```python
from build123d import *

# Parameters (mm, degrees)
BOSS_EXTRUDE1_DEPTH = 24
CUT_EXTRUDE1_DEPTH  = 29.5
SKETCH3_R           = 21
BOSS_EXTRUDE2_DEPTH = 24
CUT_EXTRUDE2_DEPTH  = 4
BOSS_EXTRUDE3_DEPTH = 11
SKETCH6_W           = 89
SKETCH6_H           = 21.5
SKETCH7_W           = 48
SKETCH7_H           = 22
BOSS_EXTRUDE4_DEPTH = 3.027047
SKETCH8_R           = 18.5
CUT_EXTRUDE3_DEPTH  = 83
CUT_EXTRUDE4_REACH  = 91
SKETCH9_R           = 1.6
SKETCH9_R_2         = 6.1
CUT_EXTRUDE5_REACH  = 125.5
SKETCH10_R          = 2.9
CUT_EXTRUDE6_REACH  = 136
SKETCH13_R          = 1.9
CUT_EXTRUDE7_DEPTH  = 27


with BuildPart() as part:
    # Sketch1 → Boss-Extrude1 (new body)
    with BuildSketch(Plane(origin=(0, 0, 0), x_dir=(1, 0, 0), z_dir=(0, 1, 0))):
        with BuildLine():
            Line((-42, 0), (-42, 11))
            Line((-42, 11), (-9.786517927, 24.087840644))
            ThreePointArc((-9.786517927, 24.087840644), (26, 0), (-9.786517927, -24.087840644))
            Line((-9.786517927, -24.087840644), (-42, -11))
            Line((-42, -11), (-42, 0))
        make_face()
    extrude(amount=BOSS_EXTRUDE1_DEPTH)

    # Sketch2 → Cut-Extrude1 (cut, symmetric)
    with BuildSketch(Plane.XY):
        Polygon((-24, 0), (26, 12), (26, 0), align=None)
    extrude(amount=CUT_EXTRUDE1_DEPTH, both=True, mode=Mode.SUBTRACT)

    # Sketch3 → Boss-Extrude2 (add)
    with BuildSketch(Plane(origin=(0, 24, 0), x_dir=(1, 0, 0), z_dir=(0, 1, 0))):
        Circle(SKETCH3_R)
    extrude(amount=-BOSS_EXTRUDE2_DEPTH)

    # Sketch4 → Cut-Extrude2 (cut)
    with BuildSketch(Plane.XZ):
        Polygon((2.829016319, 4.9), (-2.829016319, 4.9), (-5.658032638, 0), (-2.829016319, -4.9), (2.829016319, -4.9), (5.658032638, 0), align=None)
    extrude(amount=-CUT_EXTRUDE2_DEPTH, mode=Mode.SUBTRACT)

    # Sketch5 → Boss-Extrude3 (add, symmetric)
    with BuildSketch(Plane.XY):
        with BuildLine():
            ThreePointArc((-54, 24), (-78.945219608, 10.049710337), (-92.941825352, -14.869551102))
            Line((-92.941825352, -14.869551102), (-94.786517927, -22.5))
            Line((-94.786517927, -22.5), (-94.786517927, -37.075307894))
            Line((-94.786517927, -37.075307894), (-93.178015205, -46.5))
            Line((-93.178015205, -46.5), (-90, -56.5))
            Line((-90, -56.5), (-42, -56.5))
            Line((-42, -56.5), (-63.178015205, -46.5))
            Line((-63.178015205, -46.5), (-70.786517927, -37.075307894))
            Line((-70.786517927, -37.075307894), (-70.786517927, -25.075307894))
            Line((-70.786517927, -25.075307894), (-69.738862808, -20.741751748))
            ThreePointArc((-69.738862808, -20.741751748), (-62.647337683, -7.727284744), (-50, 0))
            Line((-50, 0), (-42, 0))
            Line((-42, 0), (-42, 24))
            Line((-42, 24), (-54, 24))
        make_face()
    extrude(amount=BOSS_EXTRUDE3_DEPTH, both=True)



with BuildPart() as body_2:
    # Sketch6 → Revolve1 (revolve)
    with BuildSketch(Plane.XY):
        with Locations((-53.5, -88.75)):
            Rectangle(SKETCH6_W, SKETCH6_H)
    revolve(axis=Axis((-98, -78, 0), (1, 0, 0)))


with BuildPart() as part_1:
    add(part.part)

    add(body_2.part)  # Boss-Extrude4 merges body 2
    # Sketch7 → Boss-Extrude4 (add)
    with BuildSketch(Plane.XZ.offset(56.5)):
        with Locations((-66, 0)):
            Rectangle(SKETCH7_W, SKETCH7_H)
    extrude(amount=BOSS_EXTRUDE4_DEPTH)

    # Sketch8 → Cut-Extrude3 (cut)
    with BuildSketch(Plane.ZY.offset(98)):
        with Locations((0, -78)):
            Circle(SKETCH8_R)
    extrude(amount=-CUT_EXTRUDE3_DEPTH, mode=Mode.SUBTRACT)

    # Sketch9 → Cut-Extrude4 (cut, up to next)
    with BuildSketch(Plane(origin=(-9, 0, 0), x_dir=(0, 0, -1), z_dir=(1, 0, 0)), mode=Mode.PRIVATE) as cut_extrude4_sk1:
        with Locations((15.5, -78)):
            Circle(SKETCH9_R)
    cut_extrude4_tool1 = extrude(cut_extrude4_sk1.sketch, amount=-CUT_EXTRUDE4_REACH, mode=Mode.PRIVATE) & part_1.part
    add(cut_extrude4_tool1.solids().sort_by_distance((-9, -78, -15.5))[0], mode=Mode.SUBTRACT)
    # Sketch9 → Cut-Extrude4 (cut, up to next)
    with BuildSketch(Plane(origin=(-9, 0, 0), x_dir=(0, 0, -1), z_dir=(1, 0, 0)), mode=Mode.PRIVATE) as cut_extrude4_sk2:
        with Locations((7.75, -91.423393759)):
            Circle(SKETCH9_R)
    cut_extrude4_tool2 = extrude(cut_extrude4_sk2.sketch, amount=-CUT_EXTRUDE4_REACH, mode=Mode.PRIVATE) & part_1.part
    add(cut_extrude4_tool2.solids().sort_by_distance((-9, -91.423394, -7.75))[0], mode=Mode.SUBTRACT)
    # Sketch9 → Cut-Extrude4 (cut, up to next)
    with BuildSketch(Plane(origin=(-9, 0, 0), x_dir=(0, 0, -1), z_dir=(1, 0, 0)), mode=Mode.PRIVATE) as cut_extrude4_sk3:
        with Locations((-7.75, -91.423393759)):
            Circle(SKETCH9_R)
    cut_extrude4_tool3 = extrude(cut_extrude4_sk3.sketch, amount=-CUT_EXTRUDE4_REACH, mode=Mode.PRIVATE) & part_1.part
    add(cut_extrude4_tool3.solids().sort_by_distance((-9, -91.423394, 7.75))[0], mode=Mode.SUBTRACT)
    # Sketch9 → Cut-Extrude4 (cut, up to next)
    with BuildSketch(Plane(origin=(-9, 0, 0), x_dir=(0, 0, -1), z_dir=(1, 0, 0)), mode=Mode.PRIVATE) as cut_extrude4_sk4:
        with Locations((-15.5, -78)):
            Circle(SKETCH9_R)
    cut_extrude4_tool4 = extrude(cut_extrude4_sk4.sketch, amount=-CUT_EXTRUDE4_REACH, mode=Mode.PRIVATE) & part_1.part
    add(cut_extrude4_tool4.solids().sort_by_distance((-9, -78, 15.5))[0], mode=Mode.SUBTRACT)
    # Sketch9 → Cut-Extrude4 (cut, up to next)
    with BuildSketch(Plane(origin=(-9, 0, 0), x_dir=(0, 0, -1), z_dir=(1, 0, 0)), mode=Mode.PRIVATE) as cut_extrude4_sk5:
        with Locations((-7.75, -64.576606241)):
            Circle(SKETCH9_R)
    cut_extrude4_tool5 = extrude(cut_extrude4_sk5.sketch, amount=-CUT_EXTRUDE4_REACH, mode=Mode.PRIVATE) & part_1.part
    add(cut_extrude4_tool5.solids().sort_by_distance((-9, -64.576606, 7.75))[0], mode=Mode.SUBTRACT)
    # Sketch9 → Cut-Extrude4 (cut, up to next)
    with BuildSketch(Plane(origin=(-9, 0, 0), x_dir=(0, 0, -1), z_dir=(1, 0, 0)), mode=Mode.PRIVATE) as cut_extrude4_sk6:
        with Locations((7.75, -64.576606241)):
            Circle(SKETCH9_R)
    cut_extrude4_tool6 = extrude(cut_extrude4_sk6.sketch, amount=-CUT_EXTRUDE4_REACH, mode=Mode.PRIVATE) & part_1.part
    add(cut_extrude4_tool6.solids().sort_by_distance((-9, -64.576606, -7.75))[0], mode=Mode.SUBTRACT)
    # Sketch9 → Cut-Extrude4 (cut, up to next)
    with BuildSketch(Plane(origin=(-9, 0, 0), x_dir=(0, 0, -1), z_dir=(1, 0, 0)), mode=Mode.PRIVATE) as cut_extrude4_sk7:
        with Locations((0, -85)):
            Circle(SKETCH9_R_2)
    cut_extrude4_tool7 = extrude(cut_extrude4_sk7.sketch, amount=-CUT_EXTRUDE4_REACH, mode=Mode.PRIVATE) & part_1.part
    add(cut_extrude4_tool7.solids().sort_by_distance((-9, -85, 0))[0], mode=Mode.SUBTRACT)

    # Sketch10 → Cut-Extrude5 (cut, up to next)
    with BuildSketch(Plane(origin=(0, 24, 0), x_dir=(1, 0, 0), z_dir=(0, 1, 0)), mode=Mode.PRIVATE) as cut_extrude5_sk1:
        Circle(SKETCH10_R)
    cut_extrude5_tool1 = extrude(cut_extrude5_sk1.sketch, amount=-CUT_EXTRUDE5_REACH, mode=Mode.PRIVATE) & part_1.part
    add(cut_extrude5_tool1.solids().sort_by_distance((0, 24, 0))[0], mode=Mode.SUBTRACT)

    # Sketch12 → Cut-Extrude6 (cut, up to next)
    with BuildSketch(Plane.ZY.offset(108), mode=Mode.PRIVATE) as cut_extrude6_sk1:
        Polygon((0, -14.869551102), (0, -37.075307894), (-35.009935155, -37.075307894), (-35.009935155, -113.334550455), (34.515095082, -113.334550455), (34.515095082, -14.869551102), align=None)
    cut_extrude6_tool1 = extrude(cut_extrude6_sk1.sketch, amount=-CUT_EXTRUDE6_REACH, mode=Mode.PRIVATE) & part_1.part
    add(cut_extrude6_tool1.solids().sort_by_distance((-108, -68.986865, 1.963457))[0], mode=Mode.SUBTRACT)

    # Sketch13 → Cut-Extrude7 (cut, through all)
    with BuildSketch(Plane.XY):
        with Locations((-81.960177429, -20.369551102)):
            Circle(SKETCH13_R)
        with Locations((-82.786517927, -31.575307894)):
            Circle(SKETCH13_R)
    extrude(amount=-CUT_EXTRUDE7_DEPTH, mode=Mode.SUBTRACT)


solid = part_1.part
```
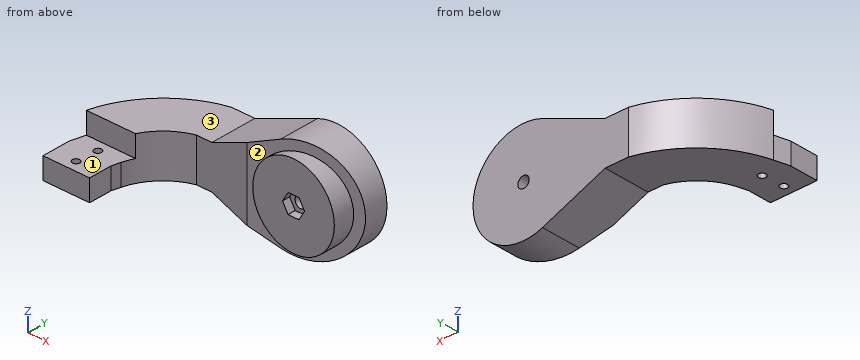
Could you check a few things on this model? Use its own coordinates, in mm. Face numbers are marked on the shaded views. A direction names the side the tool comes from. Round coordinates to 2 decimals unless told otherwise and drop trailing zeros. Loops run counter-clockwise (first coordinate to the right, second up) from the corner with the lowest first, then second, coordinate; pieces in that order, holes last. Notation, with made-up numbers: (34, 79) - (78, 79) arc R24 cw to (78, 112) - close; hole circle Ø9 at (38, 42). An arc over 180 degrees is marked (long way). Answer in a Markdown table with one row per item. Add a question column.
(1) If we section it at C-C (y = 19.5): Please give me the cut outline in (x, z).
(2) I'm going to push flat-ended pins straight in: pin 1 (13 mm diameter, centred on x = -38, z = 9, fed in from -Y); pin 2 (3.5 mm diameter, centred on y = -33, z = -4.5, fed in from +X); pin 3 (1.5 mm diameter, centred on x = -58, z = -7, fed in from +Y); pin 4 (6.5 mm diameter, centred on x = 0, z = 0, fed in from +Y). Where does each tip first touch, or does it pass through?
(3) If we section it at D-D (x = -77.5): Please give me the cut outline in (y, z), plus the area to 3 significant figures.
(4) For the marked faces 1, 2 and 3, which set-ups out of +Z, -Z, +X, -X, +Y, -Y let a thin tool reach every point of the face, with its end or its side?
(5) I need wall thicknesses on line 1 along Z through (x, y) = (0, 16); line 2 along Y through (x, z) = (-19, 2); line 3 along Z through (x, y) = (-82.5, -23.5). Which ranges of each line are inside material? Lowest first, please.
(6) If we section it at A-A (x = 0): Please give me the cut outline in (y, z), plus the area to 3 significant figures.
(7) If we section it at B-B (z = 1.5): Please give me the cut outline in (x, y), plus the area to 3 significant figures.
Model answer:
| question | item | result |
|---|---|---|
| 1 | outline | (-66.04, -11) - (-42, -11) - (-9.79, -24.09) arc R26 ccw (long way) to (-9.79, 24.09) - (-42, 11) - (-66.04, 11) - close; hole circle Ø5.8 at (0, 0) |
| 2 | pin 1 | stops at y = 0 |
| 2 | pin 2 | stops at x = -70.79 |
| 2 | pin 3 | stops at y = 23.11 |
| 2 | pin 4 | stops at y = 24 |
| 3 | outline | (-37.08, -11) - (11.44, -11) - (11.44, 11) - (-14.87, 11) - (-14.87, 0) - (-37.08, 0) - close |
| 3 | area | 823 mm² |
| 4 | face 1 | +Z, +X, -X, -Y |
| 4 | face 2 | -Y |
| 4 | face 3 | +Z, -X, +Y, -Y |
| 5 | line 1 | z = -26 to -2.9, 2.9 to 26 |
| 5 | line 2 | y = 0 to 24 |
| 5 | line 3 | z = -11 to 0 |
| 6 | outline | (0, -21) - (5.76, -21) - (5.76, -26) - (24, -26) - (24, -2.9) - (4, -2.9) - (4, -4.9) - (0, -4.9) - close; (0, 4.9) - (4, 4.9) - (4, 2.9) - (24, 2.9) - (24, 26) - (5.76, 26) - (5.76, 21) - (0, 21) - close |
| 6 | area | 1,040 mm² |
| 7 | outline | (-92.94, -14.87) - (-67.62, -14.87) arc R28.64 cw to (-50, 0) - (-24, 0) - (-20.95, 0.73) - (-20.95, 0) - (-4.79, 0) - (-4.79, 4) - (-2.48, 4) - (-2.48, 24) - (-54, 24) arc R52.71 ccw to start; (2.48, 4) - (4.79, 4) - (4.79, 0) - (20.95, 0) - (20.95, 10.79) - (25.96, 11.99) - (25.96, 24) - (2.48, 24) - close |
| 7 | area | 2,660 mm² |
